Build history of the part. All positions in model axes, mm. Face numbers are marked on the shaded views. Give positions to 0.01 mm unless a question says otherwise; leave off trailing zeros. Loops run counter-clockwise (first coordinate to the right, second up) from the corner with the lowest first, then second, coordinate; pieces in that order, holes last. Notation, with made-up numbers: M -31,50 L -3,50 A17 ccw -3,81 Z; hole C 11.25,24 d9. An arc over 180 degrees is marked long. Answer as a JSON object with one key per item and string values. Group by question number.
1. Slice it at A-A (x = 0). Give the number of separate pieces and of enclosed holes in the cut face, then the cut area to 3 significant figures.
2. Slice it at D-D (x = 24). List the corners of the cut face in (y, z) (3 decimals), then the cut area to 3 significant figures.
3. Drill centre lines: line 1 along Z through (x, y) = (0, -7.1); line 2 along Z through (x, y) = (0, -7.05); line 3 along Z through (x, y) = (5, -3). Where is each one in solid material? Low to high. Write a range as [from, to].
4. Mould opens along Z. For the marked faces 1, 2 and 3 say: released by +Z, released by -Z, zero draft, split by the parting line, or undercut.
5. Drop flat-ended pins along their axis: pin 1 Ø5 at (x, z) = (0, -44.45) entering from +Y (3 decimals); pin 2 Ø3 at (y, z) = (-9, -7) entering from -X; pin 3 Ø3 at (x, y) = (2.5, -8.5) entering from +Z. Give the stop position or say it passes through.
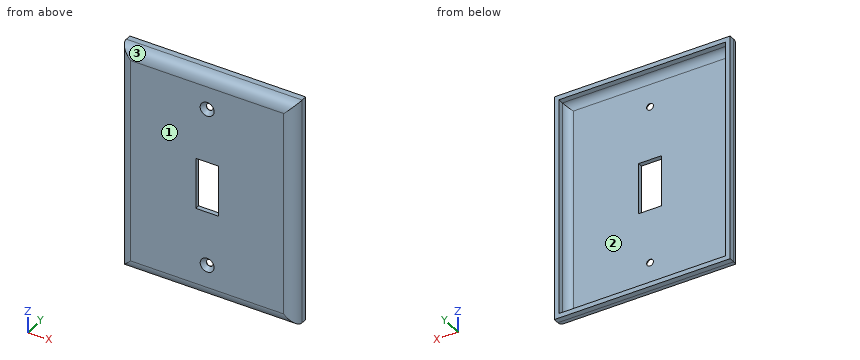
from build123d import *

# Parameters (mm, degrees)
F0_W           = 98.425
F0_H           = 127
F1_DEPTH       = 9.525
F2_R           = 6.35
F3_T           = -2.54
F4_W           = 12.7
F4_H           = 28.575
F5_DEPTH       = 9.526
F6_D           = 3.7973
F6_DEPTH       = 12.7
F6_CSINK_D     = 7.7978
F6_CSINK_ANGLE = 82
F6_TIP         = 1.1408240143


with BuildPart() as f1:
    # F0 (on Front) → F1 (new body)
    with BuildSketch(Plane.XZ):
        Rectangle(F0_W, F0_H)
    extrude(amount=F1_DEPTH)

    # F2
    f2_edges = [f1.edges().sort_by_distance(p)[0] for p in [
        (49.2125, -9.525, 0),
        (0, -9.525, 63.5),
        (-49.2125, -9.525, 0),
        (0, -9.525, -63.5),
    ]]
    fillet(f2_edges, radius=F2_R)

    # F3
    f3_openings = [f1.faces().sort_by_distance(p)[0] for p in [
        (0, 0, 0),
    ]]
    offset(amount=F3_T, openings=f3_openings)

    # F4 (on face) → F5 (cut, through all)
    with BuildSketch(Plane.XZ.offset(9.525)):
        Rectangle(F4_W, F4_H)
    extrude(amount=-F5_DEPTH, mode=Mode.SUBTRACT)

    # F6
    with Locations(Plane.XZ.offset(9.525)):
        with Locations((0, 44.45), (0, -44.45)):
            CounterSinkHole(F6_D / 2, F6_CSINK_D / 2, depth=F6_DEPTH, counter_sink_angle=F6_CSINK_ANGLE)
            with Locations((0, 0, -(F6_DEPTH + F6_TIP / 2))):  # 118° drill point
                Cone(0, F6_D / 2, F6_TIP, mode=Mode.SUBTRACT)


solid = f1.part
Established:
{
 "1": {"separate pieces": "4", "enclosed holes": "0", "area": "246 mm^2"},
 "2": {"outline": "M -9.525,-57.15 A6.35 ccw -3.175,-63.5 L 0,-63.5 L 0,-60.96 L -3.175,-60.96 A3.81 cw -6.985,-57.15 L -6.985,57.15 A3.81 cw -3.175,60.96 L 0,60.96 L 0,63.5 L -3.175,63.5 A6.35 ccw -9.525,57.15 Z", "area": "347 mm^2"},
 "3": {"line 1": "z = [-62.14, -46.35], [-42.55, -14.29], [14.29, 42.55], [46.35, 62.14]", "line 2": "z = [-62.18, -46.35], [-42.55, -14.29], [14.29, 42.55], [46.35, 62.18]", "line 3": "z = [-63.5, -60.96], [60.96, 63.5]"},
 "4": {"face 1": "zero draft", "face 2": "undercut", "face 3": "released by +Z"},
 "5": {"pin 1": "stops at y = -6.985", "pin 2": "stops at x = -47.51", "pin 3": "stops at z = 62.22"}
}
